Geometry check sheet. Reference: drawing and pictorial views, mm from the part's lowest x, y, z. Coordinates: 2 decimals unless noted, no trailing zeros. Write each loop counter-clockwise with the first axis right and the second up, starting at its lowest first coordinate (ties: lowest second). Pieces come first, ordered by that corner, then holes. Notation, with made-up numbers: (22, 88.25) - (38, 88.25) arc R11 cw to (38, 105.25) - close; hole circle Ø11 at (-33, 38). An arc over 180 degrees is marked (long way). Answer as CSV lines item,"result". Start each with the question number.
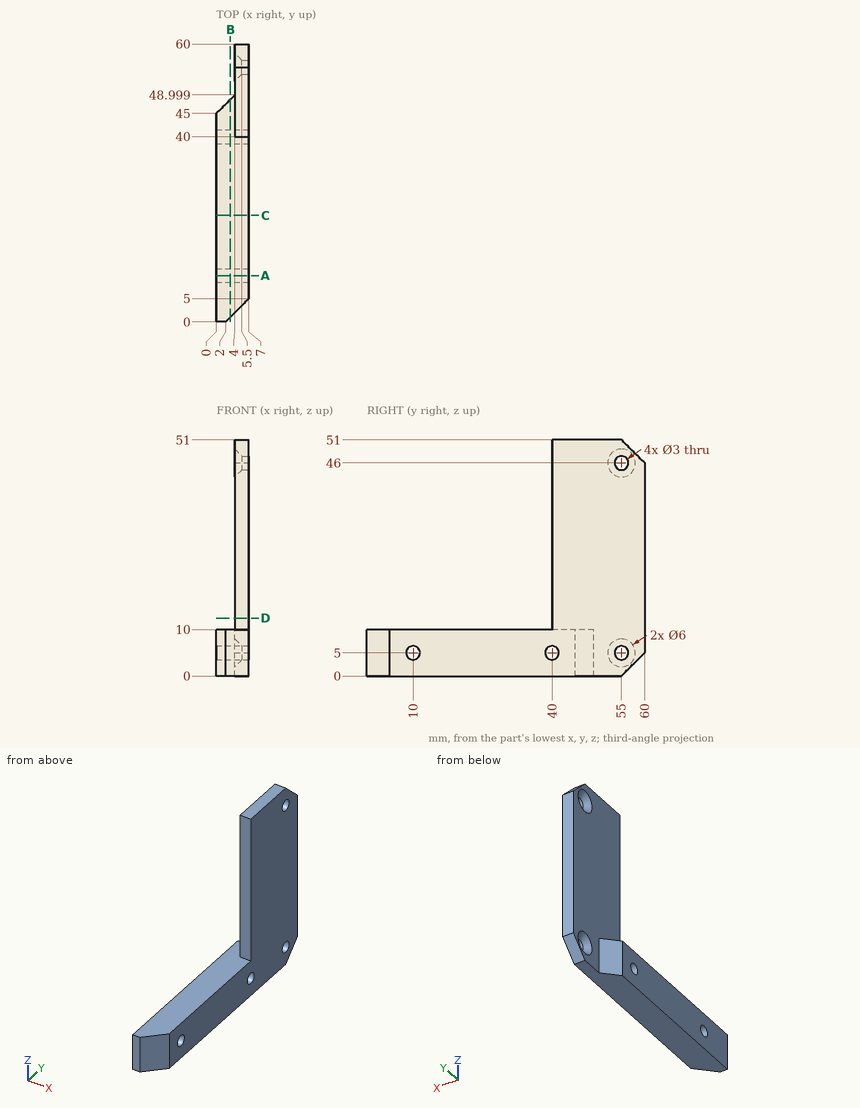
1. Cross-section at D-D (z = 12.5). Record the cut outline in (x, y), and give its area (3 significant figures).
2. Cross-section at C-C (y = 23). Record the cut outline in (x, z).
3. Cross-section at B-B (x = 3). Record the cut outline in (y, z).
4. Cross-section at A-A (y = 10). Record the cut outline in (x, z), and give its area (3 significant figures).
5. Depth check by flat-ended pin: P1, Ø22, axis at y = 52, z = 24.5, coming from the -X side; P2, Ø5, axis at y = 55, z = 5, coming from the +X side; P3, Ø2, axis at x = 2.5, y = 40, coming from the +Z side; P4, Ø5, axis at y = 55, z = 46, coming from the -X side. Enter the tip coordinate at first touch or a pass-through.
6. Scan lines: line 1 along Z through (x, y) = (5.9, 55); line 2 along Y through (x, z) = (6, 5); line 3 along Z through (x, y) = (4, 10). Record each from-to range of solid material in increasing order. Write a range as from..to.
Completed:
1,outline,"(4, 40) - (7, 40) - (7, 60) - (4, 60) - close"
1,area,"60.0 mm2"
2,outline,"(0, 0) - (7, 0) - (7, 10) - (0, 10) - close"
3,outline,"(1, 0) - (48, 0) - (48, 10) - (1, 10) - close; hole circle Ø3 at (10, 5); hole circle Ø3 at (40, 5)"
4,outline,"(0, 0) - (7, 0) - (7, 3.5) - (0, 3.5) - close; (0, 6.5) - (7, 6.5) - (7, 10) - (0, 10) - close"
4,area,"49.0 mm2"
5,P1,"stops at x = 4"
5,P2,"stops at x = 7"
5,P3,"stops at z = 10"
5,P4,"stops at x = 4.5"
6,line 1,"z = 0..3.5, 6.5..44.5, 47.5..51"
6,line 2,"y = 4..8.5, 11.5..38.5, 41.5..53.5, 56.5..60"
6,line 3,"z = 0..3.5, 6.5..10"
